Design review of the part built by this model. Coordinates are the model's own, in mm. A direction names the side the tool comes from. Round coordinates to 2 decimals unless told otherwise and drop trailing zeros. Loops run counter-clockwise (first coordinate to the right, second up) from the corner with the lowest first, then second, coordinate; pieces in that order, holes last. Notation, with made-up numbers: M 80,31 L 111,31 A9 ccw 111,46 Z; hole C -6.75,15.25 d1. An arc over 180 degrees is marked long. Use a Markdown table: item, result.
from build123d import *

# Parameters (mm, degrees)
SKETCH1_W           = 210
SKETCH1_H           = 50
SKETCH1_R           = 1.211665018
SKETCH1_R_2         = 1.165617118
SKETCH1_R_3         = 1.5
SKETCH1_R_4         = 1.517273905
SKETCH1_R_5         = 1.335614121
SKETCH1_R_6         = 1.62438417
BOSS_EXTRUDE1_DEPTH = 3.175
SKETCH2_R           = 2
CUT_EXTRUDE1_DEPTH  = 10
SKETCH3_R           = 6
SKETCH3_R_2         = 0.586995366
CUT_EXTRUDE2_DEPTH  = 57.15
CUT_EXTRUDE7_DEPTH  = 10
FILLET3_R           = 5
SKETCH11_R          = 18.5
SKETCH11_R_2        = 2
BOSS_EXTRUDE4_DEPTH = 3.175
SKETCH12_R          = 21
BOSS_EXTRUDE5_DEPTH = 3.175
SKETCH13_R          = 18.85
CUT_EXTRUDE8_DEPTH  = 3.175
BOSS_EXTRUDE6_DEPTH = 3.175
FILLET4_R           = 5
SKETCH15_R          = 1.5
CUT_EXTRUDE9_DEPTH  = 10
SKETCH16_R          = 1.5
CUT_EXTRUDE10_DEPTH = 10
SKETCH17_W          = 82.811100577
SKETCH17_H          = 66.522656387
CUT_EXTRUDE11_DEPTH = 10


with BuildPart() as part:
    # Sketch1 → Boss-Extrude1 (new body)
    with BuildSketch(Plane(origin=(0, 0, 0), x_dir=(1, 0, 0), z_dir=(0, 1, 0))):
        with Locations((105, -25)):
            Rectangle(SKETCH1_W, SKETCH1_H)
        with Locations(Location((3.489526233, -16.787661112, 0), (0, 0, 270))):
            Circle(SKETCH1_R, mode=Mode.SUBTRACT)
        with Locations(Location((34.37258772, -17.194005245, 0), (0, 0, 270))):
            Circle(SKETCH1_R_2, mode=Mode.SUBTRACT)
        with Locations(Location((37.520749958, -44.921198121, 0), (0, 0, 270))):
            Circle(SKETCH1_R_3, mode=Mode.SUBTRACT)
        with Locations(Location((168.975233936, -37.403209633, 0), (0, 0, 270))):
            Circle(SKETCH1_R_4, mode=Mode.SUBTRACT)
        with Locations(Location((116, -4.237214774, 0), (0, 0, 270))):
            Circle(SKETCH1_R_5, mode=Mode.SUBTRACT)
        with Locations(Location((12.257640281, -3.274812063, 0), (0, 0, 270))):
            Circle(SKETCH1_R_6, mode=Mode.SUBTRACT)
    extrude(amount=BOSS_EXTRUDE1_DEPTH)

    # Sketch2 → Cut-Extrude1 (cut)
    with BuildSketch(Plane(origin=(0, 3.175, 0), x_dir=(1, 0, 0), z_dir=(0, 1, 0))):
        with Locations(Location((10, -26, 0), (0, 0, 270))):
            Circle(SKETCH2_R)
        with Locations(Location((10, -42, 0), (0, 0, 270))):
            Circle(SKETCH2_R)
        with Locations(Location((26, -26, 0), (0, 0, 270))):
            Circle(SKETCH2_R)
        with Locations(Location((26, -42, 0), (0, 0, 270))):
            Circle(SKETCH2_R)
    extrude(amount=-CUT_EXTRUDE1_DEPTH, mode=Mode.SUBTRACT)

    # Sketch3 → Cut-Extrude2 (cut)
    with BuildSketch(Plane(origin=(0, 3.175, 0), x_dir=(1, 0, 0), z_dir=(0, 1, 0))):
        with Locations(Location((78.01026379, -28.1, 0), (0, 0, 270))):
            Circle(SKETCH3_R)
        with Locations(Location((145.531297368, -14, 0), (0, 0, 270))):
            Circle(SKETCH3_R)
        with Locations(Location((18, -34, 0), (0, 0, 270))):
            Circle(SKETCH3_R_2)
        with Locations(Location((202.646291021, -16, 0), (0, 0, 270))):
            Circle(SKETCH3_R)
    extrude(amount=-CUT_EXTRUDE2_DEPTH, mode=Mode.SUBTRACT)

    # Sketch10 → Cut-Extrude7 (cut)
    with BuildSketch(Plane(origin=(0, 3.175, 0), x_dir=(1, 0, 0), z_dir=(0, 1, 0))):
        Polygon((210, -27.859435908), (165.502877994, -50), (210, -50), align=None)
        Polygon((92.532613397, 0), (77.65477062, -7.402812063), (0, -7.402812063), (0, 0), align=None)
    extrude(amount=-CUT_EXTRUDE7_DEPTH, mode=Mode.SUBTRACT)

    # Fillet3
    fillet3_edges = [part.edges().sort_by_distance(p)[0] for p in [
        (210, 1.5875, 0),
        (0, 1.5875, 50),
        (92.532613397, 1.5875, 0),
        (210, 1.5875, 27.859435908),
        (165.502877994, 1.5875, 50),
        (77.65477062, 1.5875, 7.402812063),
        (0, 1.5875, 7.402812063),
    ]]
    fillet(fillet3_edges, radius=FILLET3_R)

    # Sketch11 → Boss-Extrude4 (add)
    with BuildSketch(Plane(origin=(0, 3.175, 0), x_dir=(1, 0, 0), z_dir=(0, 1, 0))):
        with Locations((18, -34)):
            Circle(SKETCH11_R)
        with Locations(Location((10, -26, 0), (0, 0, 270))):
            Circle(SKETCH11_R_2, mode=Mode.SUBTRACT)
        with Locations(Location((10, -42, 0), (0, 0, 270))):
            Circle(SKETCH11_R_2, mode=Mode.SUBTRACT)
        with Locations(Location((26, -26, 0), (0, 0, 270))):
            Circle(SKETCH11_R_2, mode=Mode.SUBTRACT)
        with Locations(Location((26, -42, 0), (0, 0, 270))):
            Circle(SKETCH11_R_2, mode=Mode.SUBTRACT)
    extrude(amount=-BOSS_EXTRUDE4_DEPTH)

    # Sketch12 → Boss-Extrude5 (add)
    with BuildSketch(Plane(origin=(0, 3.175, 0), x_dir=(1, 0, 0), z_dir=(0, 1, 0))):
        with Locations((18, -34)):
            Circle(SKETCH12_R)
    extrude(amount=-BOSS_EXTRUDE5_DEPTH)

    # Sketch13 → Cut-Extrude8 (cut)
    with BuildSketch(Plane(origin=(0, 3.175, 0), x_dir=(1, 0, 0), z_dir=(0, 1, 0))):
        with Locations(Location((18, -34, 0), (0, 0, 270))):
            Circle(SKETCH13_R)
    extrude(amount=-CUT_EXTRUDE8_DEPTH, mode=Mode.SUBTRACT)

    # Sketch14 → Boss-Extrude6 (add)
    with BuildSketch(Plane(origin=(0, 3.175, 0), x_dir=(1, 0, 0), z_dir=(0, 1, 0))):
        with BuildLine():
            Line((-35.83, -34.272812063), (-2.998227868, -34.272812063))
            ThreePointArc((-2.998227868, -34.272812063), (-2.272136238, -28.519079241), (0, -23.183346174))
            Line((0, -23.183346174), (0, -12.402812063))
            Line((0, -12.402812063), (0, -12.248529085))
            Line((0, -12.248529085), (0, 0.727187937))
            Line((0, 0.727187937), (-35.83, 0.727187937))
            Line((-35.83, 0.727187937), (-35.83, -34.272812063))
        make_face()
        with BuildLine():
            Line((0, 0.727187937), (0, -12.248529085))
            Line((0, -12.248529085), (0.002380891, -12.248529085))
            ThreePointArc((0.002380891, -12.248529085), (1.51944077, -8.813145304), (5, -7.402812063))
            Line((5, -7.402812063), (18, -7.402812063))
            Line((18, -7.402812063), (18, 0.727187937))
            Line((18, 0.727187937), (0, 0.727187937))
        make_face()
    extrude(amount=-BOSS_EXTRUDE6_DEPTH)

    # Fillet4
    fillet4_edges = [part.edges().sort_by_distance(p)[0] for p in [
        (-35.83, 1.5875, 34.272812063),
        (-35.83, 1.5875, -0.727187937),
        (18, 1.5875, -0.727187937),
    ]]
    fillet(fillet4_edges, radius=FILLET4_R)

    # Sketch15 → Cut-Extrude9 (cut)
    with BuildSketch(Plane(origin=(0, 3.175, 0), x_dir=(1, 0, 0), z_dir=(0, 1, 0))):
        with Locations(Location((122, -42.058139805, 0), (0, 0, 270))):
            Circle(SKETCH15_R)
    extrude(amount=-CUT_EXTRUDE9_DEPTH, mode=Mode.SUBTRACT)

    # Sketch16 → Cut-Extrude10 (cut)
    with BuildSketch(Plane(origin=(0, 3.175, 0), x_dir=(1, 0, 0), z_dir=(0, 1, 0))):
        with Locations(Location((12, -3.272812063, 0), (0, 0, 270))):
            Circle(SKETCH16_R)
    extrude(amount=-CUT_EXTRUDE10_DEPTH, mode=Mode.SUBTRACT)

    # Sketch17 → Cut-Extrude11 (cut)
    with BuildSketch(Plane(origin=(0, 3.175, 0), x_dir=(1, 0, 0), z_dir=(0, 1, 0))):
        with Locations((-10.47799366, -23.384449303)):
            Rectangle(SKETCH17_W, SKETCH17_H)
    extrude(amount=-CUT_EXTRUDE11_DEPTH, mode=Mode.SUBTRACT)


solid = part.part
1. Take a section at C-C on z = 14. Give the boundary of the cut face in (x, y) (3 decimals), and give its area (3 significant figures).
Check values:
| item | result |
|---|---|
| outline | M 30.928,0 L 139.531,0 L 139.531,3.175 L 30.928,3.175 Z; M 151.531,0 L 196.989,0 L 196.989,3.175 L 151.531,3.175 Z; M 208.303,0 L 210,0 L 210,3.175 L 208.303,3.175 Z |
| area | 495 mm² |
2. Machinability: for faces 1 (the face through (210, 2, 15)), 2 (the face through (54, 2, 7.403)), which of the approach directions +Z, -Z, +X, -X, +Y, -Y give a long, thin tool a straight path to every point of the face, cutting with its end or side? Answer none if there is none.
Check values:
| item | result |
|---|---|
| face 1 | +Z, -Z, +X, +Y, -Y |
| face 2 | -Z, -X, +Y, -Y |
3. The part is to be moulded in two halves that separate along X. For faces 3 (the face through (30.928, 2, 14)), 4 (the face through (38.801, 1.565, 45.703)), 5 (the face through (209.271, 1.565, 27.362)), say which applies: pulls with the +X half, pulls with the -X half, needs draft (parallel to the pull), parting line crosses it, or undercut.
Check values:
| item | result |
|---|---|
| face 3 | pulls with the -X half |
| face 4 | undercut |
| face 5 | pulls with the +X half |
4. Take a section at B-B on z = 32.5. Give the boundary of the cut face in (x, y) (3 decimals).
Check values:
| item | result |
|---|---|
| outline | M 36.79,0 L 73.931,0 L 73.931,3.175 L 36.79,3.175 Z; M 82.089,0 L 200.674,0 L 200.674,3.175 L 82.089,3.175 Z |
5. Take a section at D-D on y = 0.7. Count the separate pieces of the cut face and the enclosed holes in it, and give its area (3 significant figures).
Check values:
| item | result |
|---|---|
| separate pieces | 1 |
| enclosed holes | 8 |
| area | 7,570 mm² |
6. Take a section at A-A on x = 122. Give the boundary of the cut face in (y, z) (3 decimals).
Check values:
| item | result |
|---|---|
| outline | M 0,0 L 3.175,0 L 3.175,40.558 L 0,40.558 Z; M 0,43.558 L 3.175,43.558 L 3.175,50 L 0,50 Z |
7. Insertion check: pin 1 (2.5 mm diameter, centred on x = 122, z = 42.06, fed in from +Y); pin 2 (1 mm diameter, centred on x = 111.5, y = 2.5, fed in from +Z). Each pin has a flat end and moves straight along its axis. Give the tip position at first contact, or say it passes through.
Check values:
| item | result |
|---|---|
| pin 1 | passes through |
| pin 2 | stops at z = 50 |
8. Wall thickness on line 1 along Z through (x, y) = (145, 1.85); line 2 along X through (y, z) = (2.15, 10.5); line 3 along Z through (x, y) = (119.5, 3.05): over which ranges is each line inside the solid? List them lowest first. Write a range as from..to.
Check values:
| item | result |
|---|---|
| line 1 | z = 0..8.02, 19.98..50 |
| line 2 | x = 30.93..140.66, 150.4..200.25, 205.04..210 |
| line 3 | z = 0..50 |
